For this review, use the dimensioned drawing (mm, ordinates from the lowest corner) and the shaded views. A direction names the side the tool comes from. Round coordinates to 2 decimals unless told otherwise and drop trailing zeros. Write each loop counter-clockwise with the first axis right and the second up, starting at its lowest first coordinate (ties: lowest second). Pieces come first, ordered by that corner, then holes. Notation, with made-up numbers: M 48.25,-15.5 L 79.25,-15.5 A27 ccw 79.25,12.5 Z; hole C -20.5,83.25 d4. An arc over 180 degrees is marked long. Use one line per item in the form item = value. Start each with the question number.
Item 1: For line 1 (Z direction, x = 24.5, y = 15); line 2 (Z direction, x = 44, y = 75.5), list the stretches that pass through material, from the lowest coordinate up. Write a range as [from, to].
Item 2: For the marked faces 1, 2, 3 and 4, list the 3-axis set-ups (+Z, -Z, +X, -X, +Y, -Y) from which the entire face can be reached by the end or side of a thin tool; tool diameter is ignored.
Item 3: For P1, Ø5, axis at x = 89, z = 27.5, coming from the +Y side; P2, Ø1, axis at y = 74.5, z = 71.5, coming from the +X side; P3, Ø19.5, axis at x = 65.5, y = 76, coming from the +Z side, all flat-tipped, find the tip position at first contact; note any pin that passes through.
Item 4: Add section B-B (z = 50). State the section outline as (x, y) points.
Item 5: Add section C-C (y = 52.5). State the section outline as (x, z) points, and give its area (3 significant figures).
Item 6: Add section A-A (x = 50). State the section outline as (y, z) points, and give its area (3 significant figures).
Item 7: Add section D-D (x = 11.5). State the section outline as (y, z) points.
Item 8: Draft analysis for pull direction X (two halves, no side actions). For the marked faces 5, 6, 7 and 8, state which applies: released by +X, released by -X, zero draft, split by the parting line, or undercut.
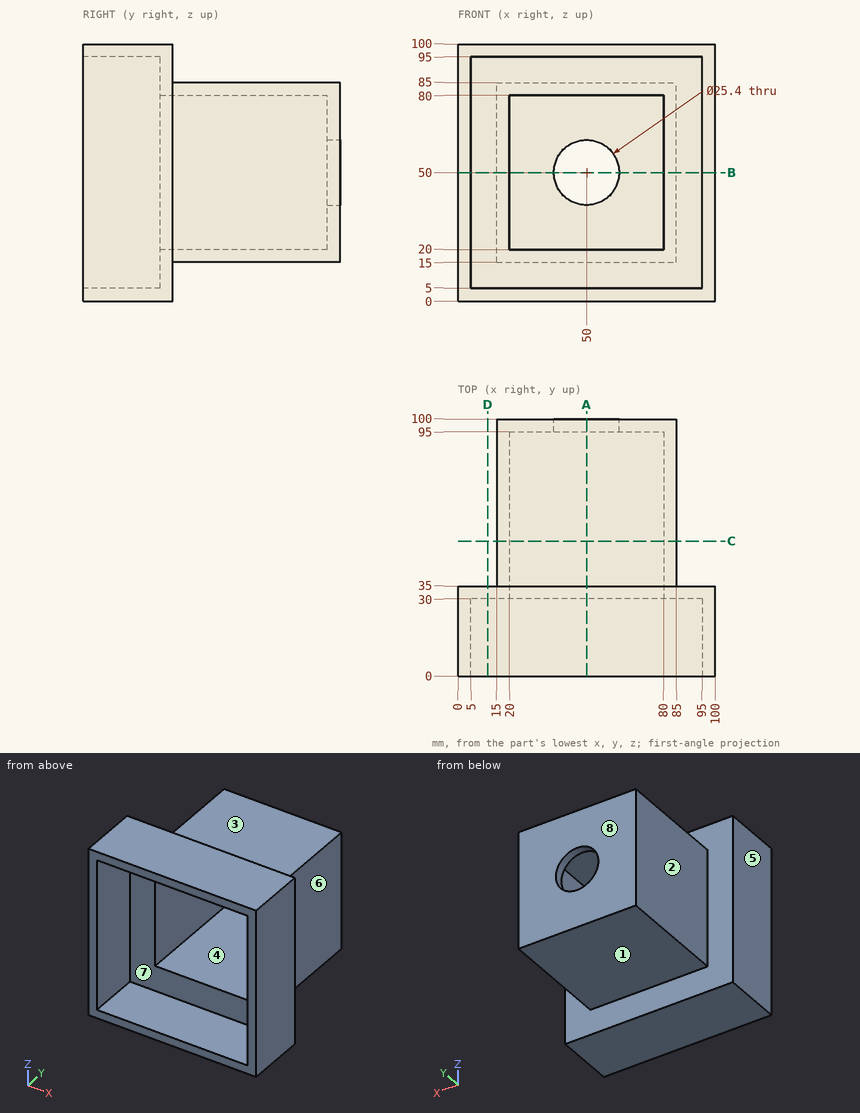
Calculated:
q1.line_1 = [0, 5], [95, 100]
q1.line_2 = [15, 20], [80, 85]
q2.face_1 = -Z, +X, -X, +Y
q2.face_2 = +Z, -Z, -X, +Y
q2.face_3 = +Z, +X, -X, +Y
q2.face_4 = -Y
q3.P1 = 35
q3.P2 = 85
q3.P3 = 85
q4.outline = M 0,0 L 5,0 L 5,30 L 20,30 L 20,95 L 37.3,95 L 37.3,100 L 15,100 L 15,35 L 0,35 Z; M 62.7,95 L 80,95 L 80,30 L 95,30 L 95,0 L 100,0 L 100,35 L 85,35 L 85,100 L 62.7,100 Z
q5.outline = M 15,15 L 85,15 L 85,85 L 15,85 Z; hole M 20,20 L 80,20 L 80,80 L 20,80 Z
q5.area = 1,300 mm^2
q6.outline = M 0,0 L 35,0 L 35,15 L 100,15 L 100,37.3 L 95,37.3 L 95,20 L 30,20 L 30,5 L 0,5 Z; M 0,95 L 30,95 L 30,80 L 95,80 L 95,62.7 L 100,62.7 L 100,85 L 35,85 L 35,100 L 0,100 Z
q6.area = 1,320 mm^2
q7.outline = M 0,0 L 35,0 L 35,100 L 0,100 L 0,95 L 30,95 L 30,5 L 0,5 Z
q8.face_5 = released by -X
q8.face_6 = released by +X
q8.face_7 = undercut
q8.face_8 = zero draft
